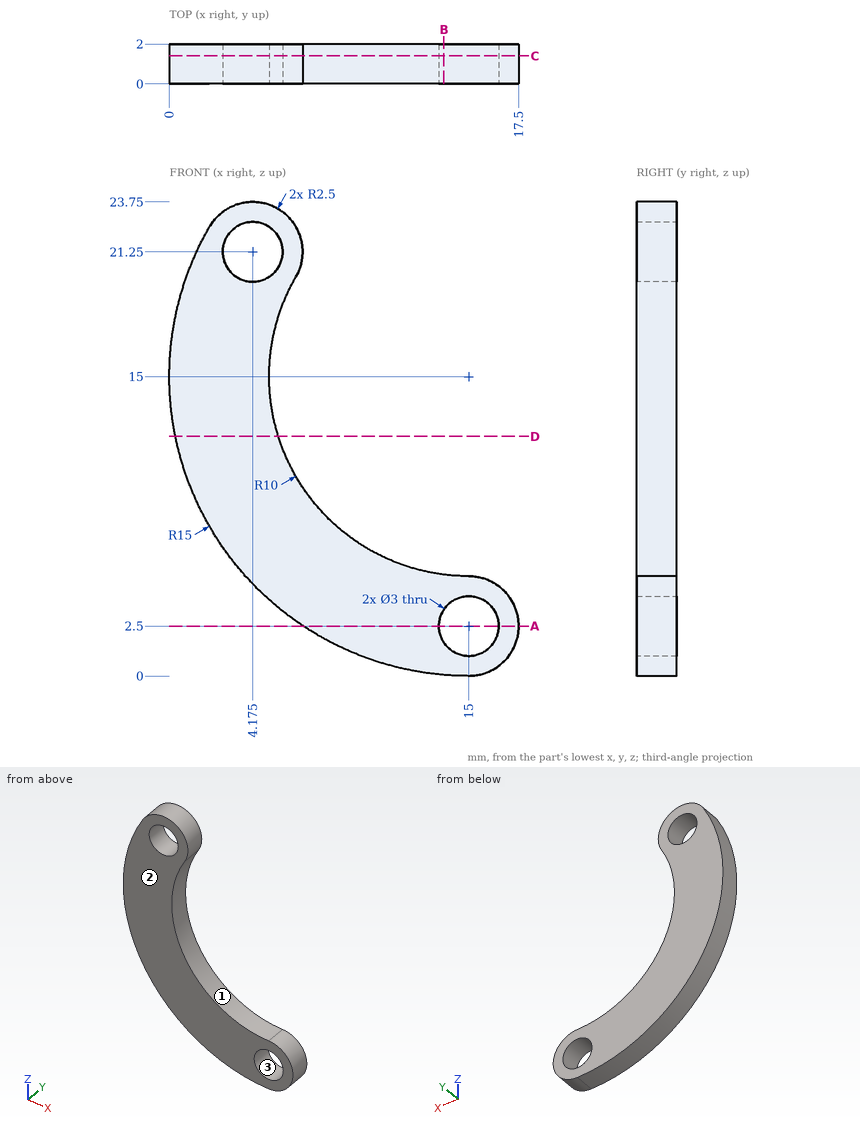
Design review of the part shown in the three views and the two pictorial views. Dimensions are in mm from the part's minimum x, y and z. Give positions to 0.01 mm unless a question says otherwise; leave off trailing zeros. Loops run counter-clockwise (first coordinate to the right, second up) from the corner with the lowest first, then second, coordinate; pieces in that order, holes last. Notation, with made-up numbers: M 31,73 L 51,73 A17 cw 51,98 Z; hole C -15,64.25 d7. An arc over 180 degrees is marked long. Put each result on its own line as item: value. Start each with the question number.
(1) Add section A-A, the plane z = 2.5. Write out the cut boundary in (x, y), then the cut area to 3 significant figures.
(2) For pin 1 (1.5 mm diameter, centred on x = 12.5, z = 6.5, fed in from -Y), flat-tipped, find the tip position at first contact; note if it passes through.
(3) The part is to be moulded in two halves that separate along X. For the marked faces 1, 2 and 3, say which applies: +X half, -X half, draft (parallel to the pull), parting line (faces both ways), or undercut.
(4) Add section B-B, the plane x = 13.75. Write out the cut boundary in (y, z).
(5) Add section D-D, the plane z = 12. Write out the cut boundary in (x, y).
(6) Add section C-C, the plane y = 1.4. Give the number of separate pieces and of enclosed holes in the cut face, then the cut area to 3 significant figures.
(7) Wall thickness on L1, parallel to Z at x = 15, y = 0.45; L2, parallel to X at y = 1.55, z = 15.25; L3, parallel to X at y = 0.1, z = 21.25 (1 decimal): over which ranges is each line inside the solid? List them lowest first.
Result:
1. outline: M 6.71,0 L 13.5,0 L 13.5,2 L 6.71,2 Z; M 16.5,0 L 17.5,0 L 17.5,2 L 16.5,2 Z
1. area: 15.6 mm^2
2. pin 1: passes through
3. face 1: +X half
3. face 2: draft
3. face 3: undercut
4. outline: M 0,0.05 L 2,0.05 L 2,1.67 L 0,1.67 Z; M 0,3.33 L 2,3.33 L 2,5.08 L 0,5.08 Z
5. outline: M 0.3,0 L 5.46,0 L 5.46,2 L 0.3,2 Z
6. separate pieces: 1
6. enclosed holes: 2
6. area: 136 mm^2
7. L1: z = 0 to 1, 4 to 5
7. L2: x = 0 to 5
7. L3: x = 1.4 to 2.7, 5.7 to 6.7
